Check sheet for the drawn part. Datum: minimum x, y, z corner. Units: mm. A direction names the side the tool comes from. Give positions to 0.01 mm unless a question says otherwise; leave off trailing zeros. Order: outer loops, then holes, each group sorted by start corner. A loop starts at its lowest first (then second) coordinate and runs counter-clockwise, first axis right, second up. Notation, with made-up numbers: (59, 31.25) -> (102, 31.25) arc R32 cw to (102, 58.25) -> close; hole circle Ø9 at (-17.75, 20.5). An arc over 180 degrees is marked (long way). Return JSON: item names as keys, results as strings. Group by question number.
(1) Tool access check on the marked faces 1, 2, 3, 4 and 5. Record the directions out of +Z, -Z, +X, -X, +Y, -Y that give a thin tool (end or side, any length) a straight path to the whole face; none if there is none.
(2) Thickness scan on line 1 along Z through (x, y) = (131, 60); line 2 along X through (y, z) = (43, 51.5); line 3 along Z through (x, y) = (15, 4.5). Record the ranges inside material, lowest first.
(3) Depth check by flat-ended pin: pin 1 Ø6 at (y, z) = (36, 74) entering from -X; pin 2 Ø4 at (x, z) = (7.5, 47.5) entering from -Y; pin 3 Ø3 at (x, y) = (87.5, 15) entering from +Z. Enter the tip coordinate at first touch or a pass-through.
(4) Cross-section at B-B on x = 70. Enter the section's corners in (y, z), then the cut area to 3 significant figures.
(5) Cross-section at C-C on y = 18.5. Enter the section's corners in (x, z), then the cut area to 3 significant figures.
(6) Cross-section at A-A on x = 131.5. Enter the section's corners in (y, z), then the cut area to 3 significant figures.
(7) Cross-section at D-D on z = 91. Enter the section's corners in (x, y), then the cut area to 3 significant figures.
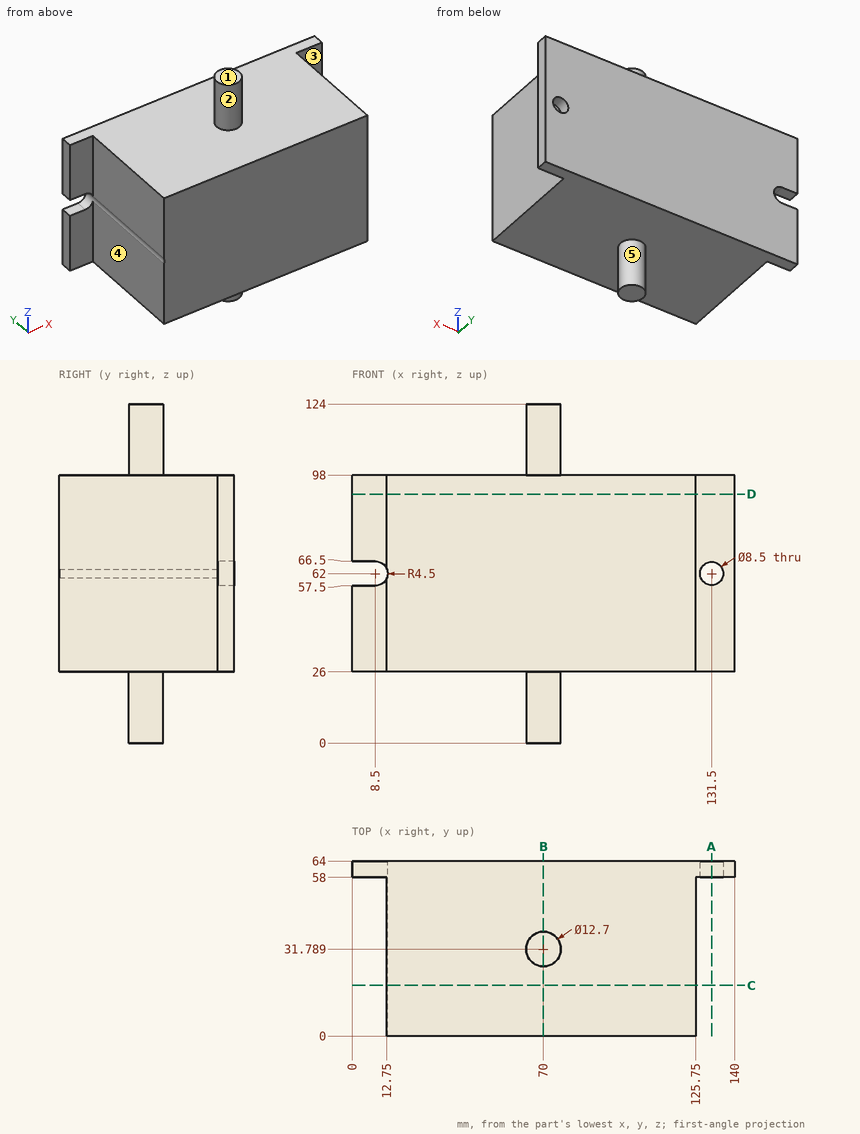
Verdict:
{
 "1": {"face 1": "+Z, +X, -X, +Y, -Y", "face 2": "+Z", "face 3": "+Z, -Z, +X, -Y", "face 4": "+Z, -Z, -X, -Y", "face 5": "-Z"},
 "2": {"line 1": "26 to 57.78, 66.22 to 98", "line 2": "12.75 to 125.75", "line 3": "26 to 98"},
 "3": {"pin 1": "x = 12.75", "pin 2": "y = 58", "pin 3": "z = 98"},
 "4": {"outline": "(0, 26) -> (25.44, 26) -> (25.44, 0) -> (38.14, 0) -> (38.14, 26) -> (64, 26) -> (64, 98) -> (38.14, 98) -> (38.14, 124) -> (25.44, 124) -> (25.44, 98) -> (0, 98) -> close", "area": "5,270 mm²"},
 "5": {"outline": "(12.75, 26) -> (125.75, 26) -> (125.75, 98) -> (12.75, 98) -> (12.75, 63.48) arc R4.5 cw to (12.75, 60.52) -> close", "area": "8,140 mm²"},
 "6": {"outline": "(58, 26) -> (64, 26) -> (64, 57.75) -> (58, 57.75) -> close; (58, 66.25) -> (64, 66.25) -> (64, 98) -> (58, 98) -> close", "area": "381 mm²"},
 "7": {"outline": "(0, 58) -> (12.75, 58) -> (12.75, 0) -> (125.75, 0) -> (125.75, 58) -> (140, 58) -> (140, 64) -> (0, 64) -> close", "area": "7,390 mm²"}
}
